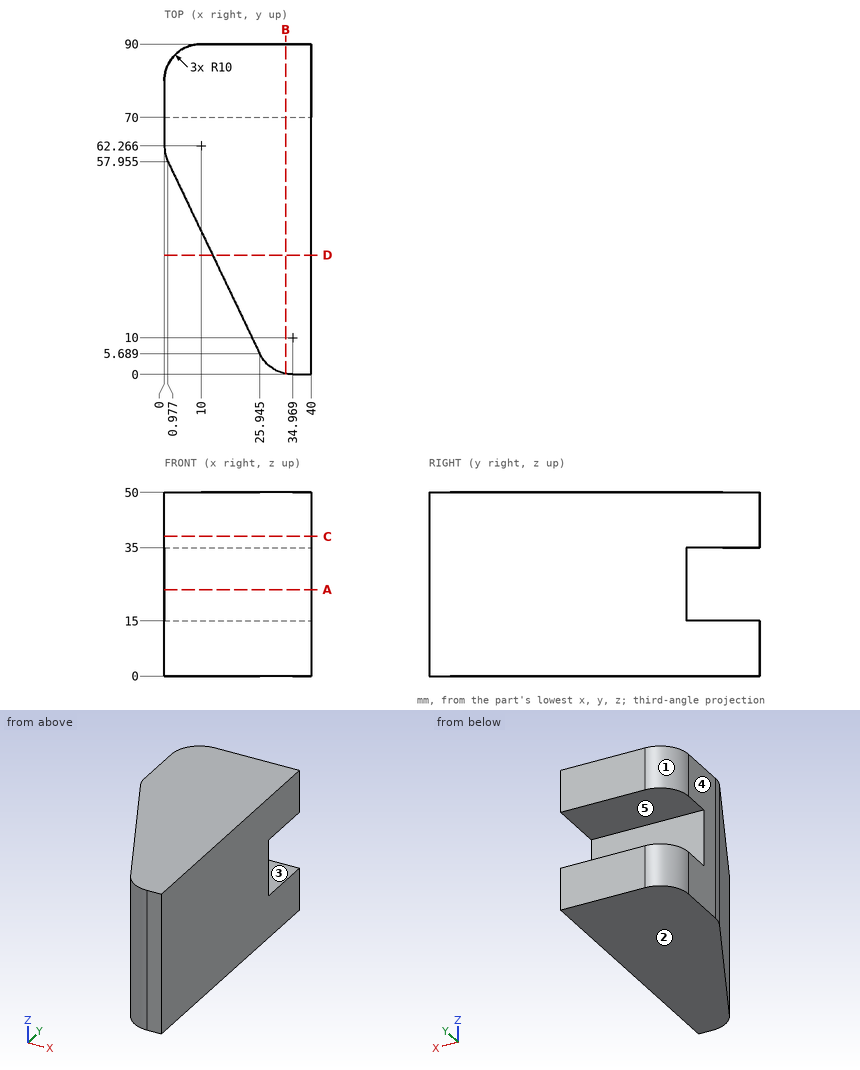
Input: dimensioned drawing with shaded views. Units: mm. Origin: part minimum x, y, z. A direction names the side the tool comes from. Coordinates: 2 decimals unless noted, no trailing zeros. Write each loop counter-clockwise with the first axis right and the second up, starting at its lowest first coordinate (ties: lowest second). Pieces come first, ordered by that corner, then holes. Notation, with made-up numbers: M 88.5,12.25 L 106.5,12.25 A15 cw 106.5,34.25 Z; hole C 87.5,1.25 d11. An arc over 180 degrees is marked long. Answer as a JSON object with one key per item and string values. Group by question number.
(1) Section A-A on z = 23.5. Output: boundary loops of the cut face in (x, y) (1 decimal).
(2) Set-up query: the marked faces 4 and 5. Return all of +Z, -Z, +X, -X, +Y, -Y with unobstructed straight access to the full face (end or side cutting, diameter ignored); none if empty.
(3) Section B-B on x = 33. Output: boundary loops of the cut face in (y, z) (1 decimal).
(4) Contact query for flat-ended pins moving along their axis: P1, Ø1.5, axis at x = 27.5, z = 31, coming from the -Y side; P2, Ø2, axis at x = 9, y = 35.5, coming from the -Z side; P3, Ø6, axis at y = 16, z = 35, coming from the -X side; P4, Ø6, axis at x = 19.5, z = 27.5, coming from the +Y side. Output: stop coordinate, or through.
(5) Section C-C on z = 38. Output: boundary loops of the cut face in (x, y) (1 decimal).
(6) Ray query, line 1 along Z through (x, y) = (20.5, 79); line 2 along Y through (x, z) = (37, 19); line 3 along Y through (x, z) = (12.5, 25) (1 decimal). Return the intervals inside material, ascending. Write a range as [from, to].
(7) Mould query, pull axis Z, two halves, no side actions, for the marked faces 1, 2 and 3. Classes: pulls with the +Z half, pulls with the -Z half, needs draft (parallel to the pull), parting line crosses it, or undercut.
(8) Section D-D on y = 32.5. Output: boundary loops of the cut face in (x, z), plus the area to 3 significant figures.
Result set:
{
 "1": {"outline": "M 0,62.3 A10 ccw 1,58 L 25.9,5.7 A10 ccw 35,0 L 40,0 L 40,70 L 0,70 Z"},
 "2": {"face 4": "+Z, -Z, -X, +Y, -Y", "face 5": "+X, -X, +Y"},
 "3": {"outline": "M 0.2,0 L 90,0 L 90,15 L 70,15 L 70,35 L 90,35 L 90,50 L 0.2,50 Z"},
 "4": {"P1": "stops at y = 2.59", "P2": "passes through", "P3": "stops at x = 19.59", "P4": "stops at y = 70"},
 "5": {"outline": "M 0,62.3 A10 ccw 1,58 L 25.9,5.7 A10 ccw 35,0 L 40,0 L 40,90 L 10,90 A10 ccw 0,80 Z"},
 "6": {"line 1": "z = [0, 15], [35, 50]", "line 2": "y = [0, 70]", "line 3": "y = [33.8, 70]"},
 "7": {"face 1": "needs draft", "face 2": "pulls with the -Z half", "face 3": "undercut"},
 "8": {"outline": "M 13.14,0 L 40,0 L 40,50 L 13.14,50 Z", "area": "1,340 mm2"}
}
